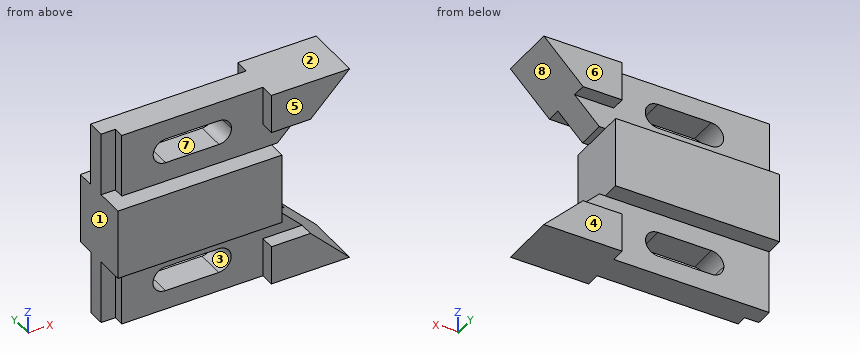
```python
from build123d import *

# Parameters (mm, degrees)
F0_W      = 104.648
F0_H      = 31.75
F1_DEPTH  = 14.224
F0_H_2    = 28.575
F2_DEPTH  = 12.7
F4_W      = 69.596
F4_H      = 6.3613896862
F5_DEPTH  = 28.575
F3_W      = 69.596
F3_H      = 6.35
F6_DEPTH  = 28.575
F7_W      = 6.35
F7_H      = 11.049
F7_W_2    = 6.3613896862
F8_DEPTH  = 52.325
F9_W      = 31.242
F9_H      = 31.75
F10_DEPTH = 28.449
F12_DEPTH = 20.575
F14_DEPTH = 26.925
F16_DEPTH = 26.925
F18_DEPTH = 20.575
F21_DEPTH = 20.575
F22_DEPTH = 20.5636103138


with BuildPart() as f1:
    # F0 (on Front) → F1 (new body, symmetric)
    with BuildSketch(Plane.XZ):
        Rectangle(F0_W, F0_H)
    extrude(amount=F1_DEPTH, both=True)

    # F0 (on Front) → F2 (join, symmetric)
    with BuildSketch(Plane.XZ):
        with Locations((0, 30.1625)):
            Rectangle(F0_W, F0_H_2)
        with Locations((0, -30.1625)):
            Rectangle(F0_W, F0_H_2)
    extrude(amount=F2_DEPTH, both=True)

    # F4 (on face) → F5 (cut)
    with BuildSketch(Plane(origin=(0, 0, -44.45), x_dir=(1, 0, 0), z_dir=(0, 0, -1))):
        Polygon((17.272, 6.35), (17.272, 12.7), (-52.324, 12.7), (-52.324, 1.524), (-45.974, 1.524), (-45.974, 6.35), align=None)
        with Locations((-17.526, -9.5193051569)):
            Rectangle(F4_W, F4_H)
    extrude(amount=-F5_DEPTH, mode=Mode.SUBTRACT)

    # F3 (on face) → F6 (cut)
    with BuildSketch(Plane.XY.offset(44.45)):
        with Locations((-17.526, 9.525)):
            Rectangle(F3_W, F3_H)
        Polygon((-45.974, -1.524), (-52.324, -1.524), (-52.324, -12.7), (17.272, -12.7), (17.272, -6.35), (-45.974, -6.35), align=None)
    extrude(amount=-F6_DEPTH, mode=Mode.SUBTRACT)

    # F7 (on Right) → F8 (cut, through all)
    with BuildSketch(Plane.YZ):
        with Locations((-9.525, 21.3995)):
            Rectangle(F7_W, F7_H)
        with Locations((9.525, 21.3995)):
            Rectangle(F7_W, F7_H)
        with Locations((9.5193051569, -21.3995)):
            Rectangle(F7_W_2, F7_H)
        with Locations((-9.525, -21.3995)):
            Rectangle(F7_W, F7_H)
    extrude(amount=F8_DEPTH, mode=Mode.SUBTRACT)

    # F9 (on face) → F10 (cut, through all)
    with BuildSketch(Plane.XZ.offset(14.224)):
        with Locations((36.703, 0)):
            Rectangle(F9_W, F9_H)
    extrude(amount=-F10_DEPTH, mode=Mode.SUBTRACT)

    # F11 (on face) → F12 (cut, through all)
    with BuildSketch(Plane.XZ.offset(6.35)):
        Polygon((23.749, -15.875), (34.798, -26.924), (52.324, -26.924), (52.324, -15.875), align=None)
    extrude(amount=-F12_DEPTH, mode=Mode.SUBTRACT)

    # F13 (on face) → F14 (cut, through all)
    with BuildSketch(Plane.XZ.offset(12.7)):
        Polygon((34.798, -26.924), (52.324, -44.45), (52.324, -26.924), align=None)
    extrude(amount=-F14_DEPTH, mode=Mode.SUBTRACT)

    # F15 (on face) → F16 (cut, through all)
    with BuildSketch(Plane(origin=(0, 12.7, 0), x_dir=(-1, 0, 0), z_dir=(0, 1, 0))):
        Polygon((-34.798, 26.924), (-52.324, 44.45), (-52.324, 26.924), align=None)
    extrude(amount=-F16_DEPTH, mode=Mode.SUBTRACT)

    # F17 (on face) → F18 (cut, through all)
    with BuildSketch(Plane(origin=(0, 6.35, 0), x_dir=(-1, 0, 0), z_dir=(0, 1, 0))):
        Polygon((-23.749, 15.875), (-34.798, 26.924), (-52.324, 26.924), (-52.324, 15.875), align=None)
    extrude(amount=-F18_DEPTH, mode=Mode.SUBTRACT)

    # F20 (on face) → F21 (cut, through all)
    with BuildSketch(Plane.XZ.offset(6.35)):
        with BuildLine():
            ThreePointArc((-26.289, 24.5745), (-22.3376873067, 26.2111873067), (-20.701, 30.1625))
            ThreePointArc((-20.701, 30.1625), (-22.3376873067, 34.1138126933), (-26.289, 35.7505))
            ThreePointArc((-26.289, 35.7505), (-31.877, 30.1625), (-26.289, 24.5745))
        make_face()
        with BuildLine():
            ThreePointArc((-26.289, 35.7505), (-22.3376873067, 34.1138126933), (-20.701, 30.1625))
            ThreePointArc((-20.701, 30.1625), (-22.3376873067, 26.2111873067), (-26.289, 24.5745))
            Line((-26.289, 24.5745), (-2.413, 24.5745))
            ThreePointArc((-2.413, 24.5745), (-8.001, 30.1625), (-2.413, 35.7505))
            Line((-2.413, 35.7505), (-26.289, 35.7505))
        make_face()
        with BuildLine():
            ThreePointArc((3.175, 30.1625), (1.5383126933, 34.1138126933), (-2.413, 35.7505))
            ThreePointArc((-2.413, 35.7505), (-8.001, 30.1625), (-2.413, 24.5745))
            ThreePointArc((-2.413, 24.5745), (1.5383126933, 26.2111873067), (3.175, 30.1625))
        make_face()
    extrude(amount=-F21_DEPTH, mode=Mode.SUBTRACT)

    # F19 (on face) → F22 (cut, through all)
    with BuildSketch(Plane(origin=(0, 6.3386103138, 0), x_dir=(-1, 0, 0), z_dir=(0, 1, 0))):
        with BuildLine():
            ThreePointArc((26.416, -35.7505), (30.3673126933, -34.1138126933), (32.004, -30.1625))
            ThreePointArc((32.004, -30.1625), (30.3673126933, -26.2111873067), (26.416, -24.5745))
            ThreePointArc((26.416, -24.5745), (20.828, -30.1625), (26.416, -35.7505))
        make_face()
        with BuildLine():
            ThreePointArc((26.416, -35.7505), (20.828, -30.1625), (26.416, -24.5745))
            Line((26.416, -24.5745), (2.54, -24.5745))
            ThreePointArc((2.54, -24.5745), (6.4913126933, -26.2111873067), (8.128, -30.1625))
            ThreePointArc((8.128, -30.1625), (6.4913126933, -34.1138126933), (2.54, -35.7505))
            Line((2.54, -35.7505), (26.416, -35.7505))
        make_face()
        with BuildLine():
            ThreePointArc((8.128, -30.1625), (6.4913126933, -26.2111873067), (2.54, -24.5745))
            ThreePointArc((2.54, -24.5745), (-3.048, -30.1625), (2.54, -35.7505))
            ThreePointArc((2.54, -35.7505), (6.4913126933, -34.1138126933), (8.128, -30.1625))
        make_face()
    extrude(amount=-F22_DEPTH, mode=Mode.SUBTRACT)


solid = f1.part
```
The listing builds one solid part. Answer for the finished solid, in the listing's coordinates (mm). Face numbers are marked on the shaded views. A direction names the side the tool comes from. Round coordinates to 2 decimals unless told otherwise and drop trailing zeros. Loops run counter-clockwise (first coordinate to the right, second up) from the corner with the lowest first, then second, coordinate; pieces in that order, holes last. Notation, with made-up numbers: (-1, 37.5) - (32, 37.5) arc R20 cw to (32, 52.5) - close; hole circle Ø6 at (-19.75, 82). An arc over 180 degrees is marked (long way). Use one line per item in the form item = value. Start each with the question number.
1. The part is cut by section B-B on x = 14. Determine the outline of the cut face in (y, z) (3 decimals), then the cut area to 3 significant figures.
2. The part is cut by section A-A on y = -7.5. Determine the outline of the cut face in (x, z) (3 decimals), then the cut area to 3 significant figures.
3. For a pull along Z with two mould halves and no side action, classify the marked faces 1, 2 and 3 as pulls with the +Z half, pulls with the -Z half, needs draft (parallel to the pull), parting line crosses it, or undercut.
4. The part is cut by section C-C on x = -8.5. Give the number of separate pieces and of enclosed holes in the cut face, then the cut area to 3 significant figures.
5. A tool of negligible diameter and unlimited length cuts with its end or side. For the marked faces 4, 5, 6, 7 and 8, from which of +Z, -Z, +X, -X, +Y, -Y can it reach the whole face along a straight path? Write none if from no direction.
6. Consider line 1 (Z direction, x = -13, y = -5.75); line 2 (Y direction, x = -45, z = -27.5); line 3 (Y direction, x = 25.5, z = 32.5). Determine where each line is inside the solid, lowest interval first. Write a range as [from, to].
7. Given pin 1 Ø4 at (x, z) = (-12, 21) entering from -Y; pin 2 Ø23 at (x, z) = (-24.5, 34.5) entering from +Y; pin 3 Ø6 at (y, z) = (-7, -20.5) entering from -X, each flat-ended and moving along its own axis, determine where each tip first touches the part or whether it passes through.
Geometry check:
q1.outline = (-14.224, -15.875) - (-6.35, -15.875) - (-6.35, -44.45) - (6.339, -44.45) - (6.339, -15.875) - (14.224, -15.875) - (14.224, 15.875) - (6.35, 15.875) - (6.35, 44.45) - (-6.35, 44.45) - (-6.35, 15.875) - (-14.224, 15.875) - close
q1.area = 1,630 mm^2
q2.outline = (-52.324, -15.875) - (21.082, -15.875) - (21.082, 15.875) - (-52.324, 15.875) - close; (17.272, -44.45) - (52.324, -44.45) - (34.798, -26.924) - (17.272, -26.924) - close; (17.272, 26.924) - (34.798, 26.924) - (52.324, 44.45) - (17.272, 44.45) - close
q2.area = 3,250 mm^2
q3.face_1 = needs draft
q3.face_2 = pulls with the +Z half
q3.face_3 = undercut
q4.separate_pieces = 3
q4.enclosed_holes = 0
q4.area = 1,340 mm^2
q5.face_4 = -Z, +X, -X, +Y
q5.face_5 = +Z, +X, -X, -Y
q5.face_6 = +Z, +X, -X, +Y
q5.face_7 = +Y, -Y
q5.face_8 = +X, +Y, -Y
q6.line_1 = [-44.45, -35.75], [-24.57, 24.57], [35.75, 44.45]
q6.line_2 = [-6.35, 6.34]
q6.line_3 = [-12.7, 12.7]
q7.pin_1 = -6.35
q7.pin_2 = 6.35
q7.pin_3 = -45.97
